```python
from build123d import *

# Parameters (mm, degrees)
F0_W     = 38.1
F0_H     = 31.75
F1_DEPTH = 25.4
F2_W     = 25.3788903356
F2_H     = 12.7
F3_DEPTH = 25.4
F4_DEPTH = 25.4
F5_DEPTH = 25.4
F6_DEPTH = 25.4


with BuildPart() as f1:
    # F0 (on Front) → F1 (new body)
    with BuildSketch(Plane.XZ):
        with Locations((19.05, 15.875)):
            Rectangle(F0_W, F0_H)
    extrude(amount=F1_DEPTH)

    # F2 (on Right) → F3 (cut)
    with BuildSketch(Plane.YZ):
        with Locations((-12.6894451678, 6.35)):
            Rectangle(F2_W, F2_H)
    extrude(amount=F3_DEPTH, mode=Mode.SUBTRACT)

    # F4 (add): a face of the model
    f4_faces = [f1.faces().sort_by_distance(p)[0] for p in [
        (12.7, -25.3788903356, 6.35),
    ]]
    extrude(f4_faces, amount=F4_DEPTH)

    # F5 (cut): a face of the model
    f5_faces = [f1.faces().sort_by_distance(p)[0] for p in [
        (12.7, 0.0211096644, 6.35),
    ]]
    extrude(f5_faces, amount=-F5_DEPTH, mode=Mode.SUBTRACT)

    # F6 (cut): a face of the model
    f6_faces = [f1.faces().sort_by_distance(p)[0] for p in [
        (12.7, -25.3788903356, 6.35),
    ]]
    extrude(f6_faces, amount=-F6_DEPTH, mode=Mode.SUBTRACT)


solid = f1.part
```
Verification items for the finished model (mm, model axes). A direction names the side the tool comes from. Coordinates: 2 decimals unless noted, no trailing zeros. Loops run counter-clockwise (first coordinate to the right, second up) from the corner with the lowest first, then second, coordinate; pieces in that order, holes last. Notation, with made-up numbers: (45, 33) - (67, 33) arc R26 ccw to (67, 62) - close; hole circle Ø10 at (56, 16.5). An arc over 180 degrees is marked (long way). Answer as a JSON object with one key per item and string values.
(1) Access from +Z, -Z, +X, -X, +Y, -Y to the whole of each face (thin tool, end or side, straight path). Record for faces 1 (the flat face through (23, -25.4, 20)), 2 (the flat face through (25.4, -13, 6)).
Response:
{"face 1": "+Z, -Z, +X, -X, -Y", "face 2": "-Z, -X, +Y, -Y"}
(2) Go/stop test with flat-tipped pins: pin 1 Ø12.5 at (x, y) = (13, -17.5) entering from -Z; pin 2 Ø14 at (y, z) = (-11, 5.5) entering from -X. Record where each tip stops, or that it passes through.
Response:
{"pin 1": "stops at z = 12.7", "pin 2": "stops at x = 25.4"}
(3) Cross-section at B-B, the plane z = 6. Record the boundary of the cut face in (x, y).
Response:
{"outline": "(25.4, -25.4) - (38.1, -25.4) - (38.1, 0) - (25.4, 0) - close"}
(4) Scan lines: line 1 along Z through (x, y) = (2.5, -13.5); line 2 along X through (y, z) = (-15.75, 5). Record each from-to range of solid material in increasing order.
Response:
{"line 1": "z = 12.7 to 31.75", "line 2": "x = 25.4 to 38.1"}
(5) Cross-section at A-A, the plane y = -21.75. Record the boundary of the cut face in (x, z), then the cut area to 3 significant figures.
Response:
{"outline": "(0, 12.7) - (25.4, 12.7) - (25.4, 0) - (38.1, 0) - (38.1, 31.75) - (0, 31.75) - close", "area": "887 mm²"}
(6) Cross-section at C-C, the plane x = 22. Record the boundary of the cut face in (y, z).
Response:
{"outline": "(-25.4, 12.7) - (0, 12.7) - (0, 31.75) - (-25.4, 31.75) - close"}
